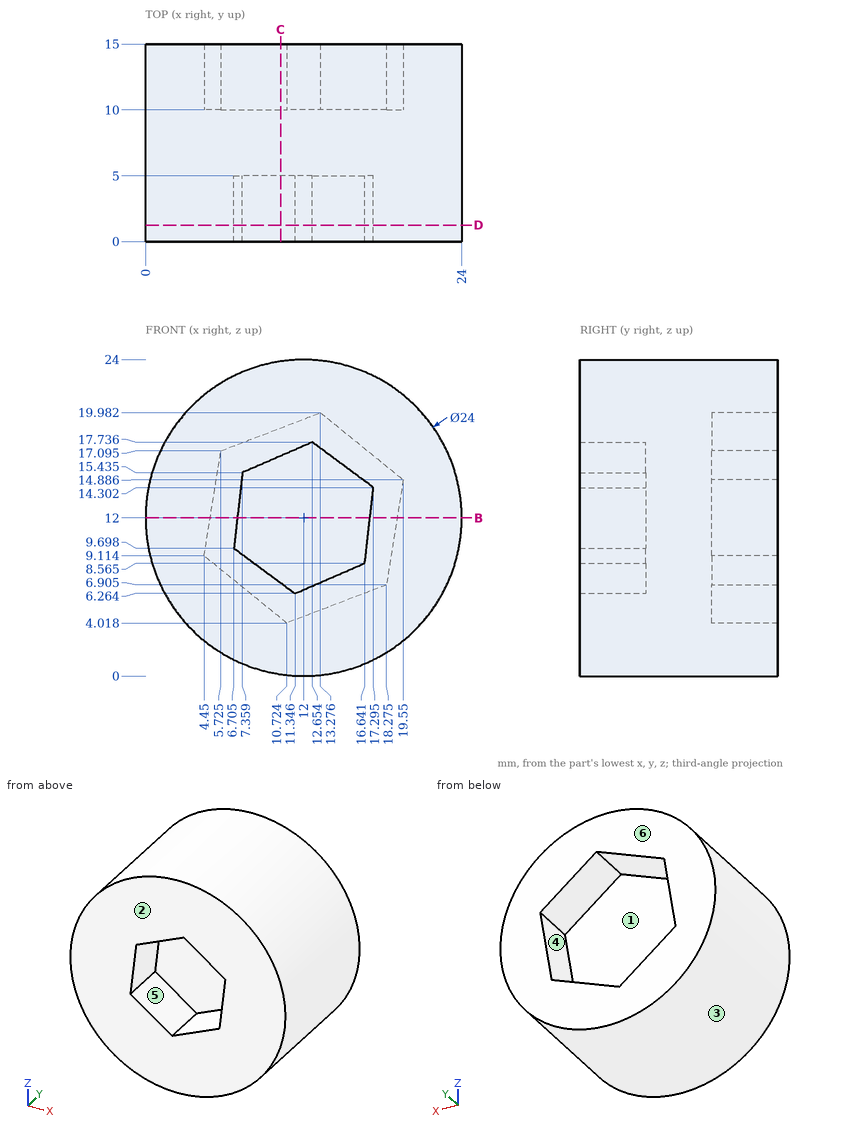
Print and shaded views of the part. All mm, measured from the part's lowest x, y and z. A direction names the side the tool comes from. Round coordinates to 2 decimals unless told otherwise and drop trailing zeros. Write each loop counter-clockwise with the first axis right and the second up, starting at its lowest first coordinate (ties: lowest second). Pieces come first, ordered by that corner, then holes. Notation, with made-up numbers: (80.5, 72.5) -> (102.5, 72.5) arc R13 ccw to (102.5, 76.5) -> close; hole circle Ø8 at (-25, 51.5). An arc over 180 degrees is marked (long way). Return JSON: item names as keys, results as strings. Group by question number.
Q1. Which spindle directions (+Z, -Z, +X, -X, +Y, -Y) get a long thin tool onto all of the face, cutting with end or side? Do the marked faces 4, 5 and 6. Say none if no direction does.
Q2. Probe L1, parallel to Y at x = 5.5, z = 12.25; L2, parallel to Y at x = 9, z = 16; L3, parallel to X at y = 13.75, z = 16.5 (1 decimal). List the from-to ranges inside material, lowest first. Write a range as [from, to].
Q3. Mould opens along Z. For the marked faces 1, 2 and 3 say: pulls with the +Z half, pulls with the -Z half, needs draft (parallel to the pull), parting line crosses it, or undercut.
Q4. Pin check, flat tips, straight feed: pin 1 (4 mm diameter, centred on y = 3.5, z = 9.5, fed in from +X); pin 2 (5 mm diameter, centred on x = 2.5, y = 6.5, fed in from -Z); pin 3 (5 mm diameter, centred on y = 4.5, z = 20.5, fed in from -X); pin 4 (8.5 mm diameter, centred on x = 11.5, z = 9, fed in from -Y). Stop position of each tip, or through.
Q5. Saw through at B-B on z = 12. Write the cut outline in (x, y).
Q6. Saw through at C-C on x = 10.25. Write the cut outline in (y, z) (1 decimal).
Q7. Saw through at D-D on y = 1.25. Write the cut outline in (x, z) (1 decimal), plus the area to 3 significant figures.
Answer:
{
 "1": {"face 4": "+Y", "face 5": "-Y", "face 6": "+Z, -Z, +X, -X, +Y"},
 "2": {"L1": "[0, 10]", "L2": "[5, 10]", "L3": "[0.9, 5.6], [17.6, 23.1]"},
 "3": {"face 1": "undercut", "face 2": "needs draft", "face 3": "parting line crosses it"},
 "4": {"pin 1": "x = 23.99", "pin 2": "z = 2.25", "pin 3": "x = 1.61", "pin 4": "y = 0"},
 "5": {"outline": "(0, 0) -> (6.97, 0) -> (6.97, 5) -> (17.03, 5) -> (17.03, 0) -> (24, 0) -> (24, 15) -> (19.09, 15) -> (19.09, 10) -> (4.91, 10) -> (4.91, 15) -> (0, 15) -> close"},
 "6": {"outline": "(0, 0.1) -> (15, 0.1) -> (15, 4.4) -> (10, 4.4) -> (10, 18.8) -> (15, 18.8) -> (15, 23.9) -> (0, 23.9) -> (0, 16.7) -> (5, 16.7) -> (5, 7.1) -> (0, 7.1) -> close"},
 "7": {"outline": "circle Ø24 at (12, 12); hole (6.7, 9.7) -> (11.3, 6.3) -> (16.6, 8.6) -> (17.3, 14.3) -> (12.7, 17.7) -> (7.4, 15.4) -> close", "area": "366 mm2"}
}
